Read the model definition and answer for the solid it produces. Units are mm, in the model's axes. Face numbers are marked on the shaded views. Coordinates: 2 decimals unless noted, no trailing zeros. Write each loop counter-clockwise with the first axis right and the second up, starting at its lowest first coordinate (ties: lowest second). Pieces come first, ordered by that corner, then holes. Notation, with made-up numbers: M 18,35.5 L 35,35.5 A27 cw 35,52.5 Z; hole C 64.25,1.25 d5. An arc over 180 degrees is marked long. Write item = value, one per line.
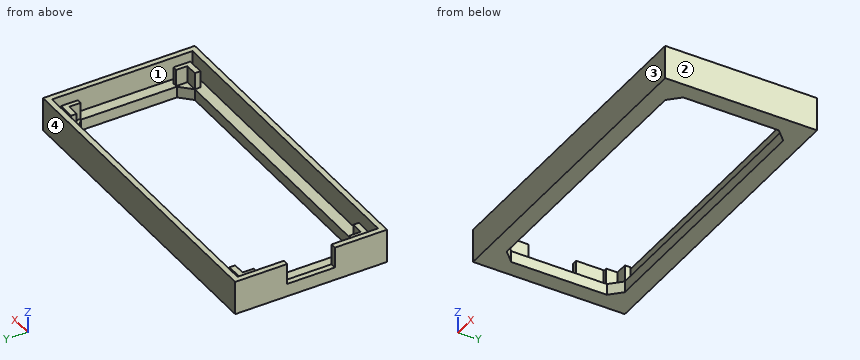
from build123d import *

# Parameters (mm, degrees)
SKETCH_W                = 57
SKETCH_H                = 27
PAD_DEPTH               = 2
PAD001_DEPTH            = 3
PAD001_MIRRORED_2_DEPTH = 3
POCKET_DEPTH            = 2
SKETCH003_W             = 57
SKETCH003_H             = 27
SKETCH003_W_2           = 55
SKETCH003_H_2           = 25
PAD002_DEPTH            = 4
SKETCH004_W             = 1
SKETCH004_H             = 8.5
POCKET001_DEPTH         = 3.7


with BuildPart() as part:
    # Sketch → Pad (new body)
    with BuildSketch(Plane.XY):
        Rectangle(SKETCH_W, SKETCH_H)
    extrude(amount=PAD_DEPTH)

    # Sketch001 (on Face6 of Pad) → Pad001 (join)
    with BuildSketch(Plane.XY.offset(2)):
        Polygon((-26.5, 11.5), (-23.5, 11.5), (-23.5, 10.5), (-25.7, 10.5), (-25.7, 8.5), (-26.5, 8.5), align=None)
    pad001 = extrude(amount=PAD001_DEPTH)

    # Sketch001 Mirrored 2 → Pad001 Mirrored 2 (add)
    with BuildSketch(Plane(origin=(0, 0, 2), x_dir=(-1, 0, 0), z_dir=(0, 0, -1))):
        Polygon((-26.5, 11.5), (-23.5, 11.5), (-23.5, 10.5), (-25.7, 10.5), (-25.7, 8.5), (-26.5, 8.5), align=None)
    pad001_mirrored_2 = extrude(amount=-PAD001_MIRRORED_2_DEPTH)

    # Mirrored001: Pad001, Pad001 Mirrored 2 across Sketch001 H_Axis
    add(pad001.mirror(Plane(origin=(0, 0, 2), x_dir=(0, 0, 1), z_dir=(0, 1, 0))))
    add(pad001_mirrored_2.mirror(Plane(origin=(0, 0, 2), x_dir=(0, 0, 1), z_dir=(0, 1, 0))))

    # Sketch002 (on Face5 of MultiTransform) → Pocket (cut)
    with BuildSketch(Plane.XY.offset(2)):
        Polygon((23.5, 10.5), (25.5, 8.5), (25.5, -8.5), (23.5, -10.5), (-23.5, -10.5), (-25.5, -8.5), (-25.5, 8.5), (-23.5, 10.5), align=None)
    extrude(amount=-POCKET_DEPTH, mode=Mode.SUBTRACT)

    # Sketch003 (on Face5 of Pocket) → Pad002 (join)
    with BuildSketch(Plane.XY.offset(2)):
        Rectangle(SKETCH003_W, SKETCH003_H)
        Rectangle(SKETCH003_W_2, SKETCH003_H_2, mode=Mode.SUBTRACT)
    extrude(amount=PAD002_DEPTH)

    # Sketch004 (on Face17 of Pad002) → Pocket001 (cut)
    with BuildSketch(Plane.XY.offset(6)):
        with Locations((-28, 0)):
            Rectangle(SKETCH004_W, SKETCH004_H)
    extrude(amount=-POCKET001_DEPTH, mode=Mode.SUBTRACT)


solid = part.part
Item 1: Find section C-C (z = 1.2). Determine the outline of the cut face in (x, y).
Worked answers:
outline = M -28.5,-13.5 L 28.5,-13.5 L 28.5,13.5 L -28.5,13.5 Z; hole M -25.5,-8.5 L -23.5,-10.5 L 23.5,-10.5 L 25.5,-8.5 L 25.5,8.5 L 23.5,10.5 L -23.5,10.5 L -25.5,8.5 Z
Item 2: Find section A-A (x = 14). Determine the outline of the cut face in (y, z), and give its area (3 significant figures).
Worked answers:
outline = M -13.5,0 L -10.5,0 L -10.5,2 L -12.5,2 L -12.5,6 L -13.5,6 Z; M 10.5,0 L 13.5,0 L 13.5,6 L 12.5,6 L 12.5,2 L 10.5,2 Z
area = 20.0 mm²
Item 3: Find section D-D (z = 4.1). State how many separate pieces and enclosed holes the cut face has, and give its area (3 significant figures).
Worked answers:
separate_pieces = 5
enclosed_holes = 0
area = 174 mm²
Item 4: For a pull along Y with two mould halves and no side action, classify the marked faces 1, 2, 3 and 4 as released by +Y, released by -Y, zero draft, split by the parting line, or undercut.
Worked answers:
face_1 = undercut
face_2 = zero draft
face_3 = released by -Y
face_4 = released by +Y
Item 5: Flat-ended cylindrical pins translate along their axes: pin 1 (2.5 mm diameter, centred on x = 24.5, y = -10.5, fed in from +Z); pin 2 (1.5 mm diameter, centred on x = -24.5, y = -9.5, fed in from +Z). Find the tip coordinate at first contact, or state that the pin passes through.
Worked answers:
pin_1 = 5
pin_2 = 2
Item 6: Consider line 1 along Y through (x, z) = (-25.5, 4.9); line 2 along Y through (x, z) = (3.5, 0.3); line 3 along X through (y, z) = (10.75, 2.9). Determine where each line is inside the solid, lowest interval first. Write a range as from..to.
Worked answers:
line_1 = -13.5..-12.5, -11.5..-10.5, 10.5..11.5, 12.5..13.5
line_2 = -13.5..-10.5, 10.5..13.5
line_3 = -28.5..-27.5, -26.5..-23.5, 23.5..26.5, 27.5..28.5
Item 7: Find section B-B (y = -7.75). Determine the outline of the cut face in (x, z), and give its area (3 significant figures).
Worked answers:
outline = M -28.5,0 L -25.5,0 L -25.5,2 L -27.5,2 L -27.5,6 L -28.5,6 Z; M 25.5,0 L 28.5,0 L 28.5,6 L 27.5,6 L 27.5,2 L 25.5,2 Z
area = 20.0 mm²
